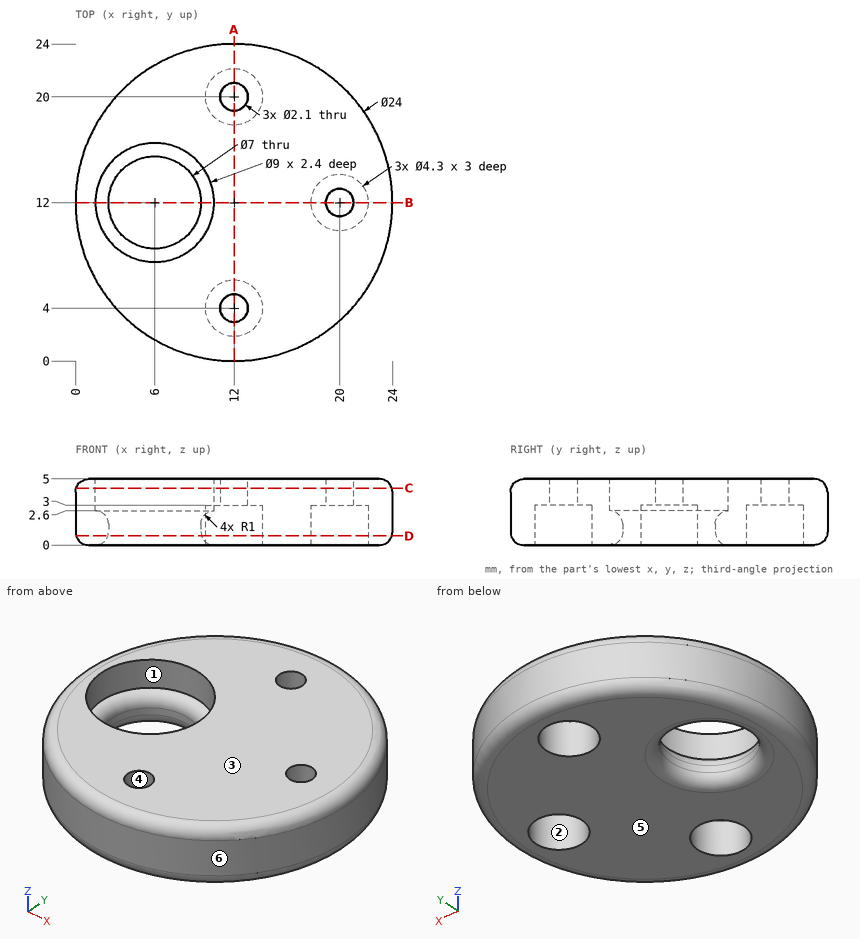
Study the drawing (mm; zero at the part's minimum x, y, z) and answer. A direction names the side the tool comes from. Round coordinates to 2 decimals unless told otherwise and drop trailing zeros. Order: outer loops, then holes, each group sorted by start corner. A loop starts at its lowest first (then second) coordinate and runs counter-clockwise, first axis right, second up. Notation, with made-up numbers: (-38.75, 13) - (-4.75, 13) arc R19 ccw to (-4.75, 39) - close; hole circle Ø5 at (49.5, 13). An arc over 180 degrees is marked (long way). Use one line per item in the form item = value. Start each with the question number.
(1) Flat-ended cylindrical pins translate along their axes: pin 1 Ø1 at (x, z) = (18.5, 2.5) entering from +Y; pin 2 Ø5 at (x, y) = (13, 4) entering from +Z; pin 3 Ø1.3 at (x, y) = (12, 20.5) entering from -Z; pin 4 Ø3 at (x, z) = (18.5, 2.5) entering from +Y. Find the tip coordinate at first contact, or state that the pin passes through.
(2) For the marked faces 1, 2 and 3, determine the directions among +Z, -Z, +X, -X, +Y, -Y from which every point of the face is accessible in a straight line to the end or side of a thin tool.
(3) Find the intervals of material crossed by line 1 along X through (y, z) = (13.5, 1.2); line 2 along Y through (x, z) = (12, 0.6); line 3 along Z through (x, y) = (11, 1), in increasing order. Write a range as from..to.
(4) The part is cut by section D-D (z = 0.7). Give the vertices of the cut face in (x, y).
(5) The part is cut by section B-B (y = 12). Count the separate pieces of the cut face and the enclosed holes in it, then the cut area to 3 significant figures.
(6) Determine the mould class of the marked faces 4, 5 and 6 for opening direction Y: +Y half, -Y half, draft (parallel to the pull), parting line (faces both ways), or undercut.
(7) The part is cut by section A-A (x = 12). Give the vertices of the cut face in (y, z).
(8) The part is cut by section C-C (z = 4.3). Give the vertices of the cut face in (x, y), then the cut area to 3 significant figures.
Checked values:
q1.pin_1 = 22.39
q1.pin_2 = 5
q1.pin_3 = 3
q1.pin_4 = 22.91
q2.face_1 = +Z
q2.face_2 = -Z
q2.face_3 = +Z, +X, -X, +Y, -Y
q3.line_1 = 0.09..2.84, 9.16..18.46, 21.54..23.91
q3.line_2 = 0.08..1.85, 6.15..17.85, 22.15..23.92
q3.line_3 = 0..5
q4.outline = circle Ø23.91 at (12, 12); hole circle Ø7.09 at (6, 12); hole circle Ø4.3 at (12, 4); hole circle Ø4.3 at (12, 20); hole circle Ø4.3 at (20, 12)
q5.separate_pieces = 3
q5.enclosed_holes = 0
q5.area = 61.4 mm^2
q6.face_4 = undercut
q6.face_5 = draft
q6.face_6 = parting line
q7.outline = (0, 1) arc R1 ccw to (1, 0) - (1.85, 0) - (1.85, 3) - (2.95, 3) - (2.95, 5) - (1, 5) arc R1 ccw to (0, 4) - close; (5.05, 3) - (6.15, 3) - (6.15, 0) - (17.85, 0) - (17.85, 3) - (18.95, 3) - (18.95, 5) - (5.05, 5) - close; (21.05, 3) - (22.15, 3) - (22.15, 0) - (23, 0) arc R1 ccw to (24, 1) - (24, 4) arc R1 ccw to (23, 5) - (21.05, 5) - close
q8.outline = circle Ø23.91 at (12, 12); hole circle Ø9 at (6, 12); hole circle Ø2.1 at (12, 4); hole circle Ø2.1 at (12, 20); hole circle Ø2.1 at (20, 12)
q8.area = 375 mm^2
